from build123d import *

# Parameters (mm, degrees)
ESQUISSE1_W             = 29.88
ESQUISSE1_H             = 30
ESQUISSE1_W_2           = 30
BOSS_EXTRU_1_DEPTH      = 3
ENL_V_MAT_EXTRU_1_DEPTH = 3


with BuildPart() as part:
    # Esquisse1 → Boss.-Extru.1 (new body)
    with BuildSketch(Plane(origin=(0, 0, 0), x_dir=(0, 0, -1), z_dir=(1, 0, 0))):
        with Locations((29.757813765, -25.688259109)):
            Rectangle(ESQUISSE1_W, ESQUISSE1_H)
        with Locations((-0.182186235, -25.688259109)):
            Rectangle(ESQUISSE1_W_2, ESQUISSE1_H)
        with Locations((-0.182186235, 4.311740891)):
            Rectangle(ESQUISSE1_W_2, ESQUISSE1_H)
    extrude(amount=BOSS_EXTRU_1_DEPTH)

    # Esquisse2 → Enlèv. mat.-Extru.1 (cut)
    with BuildSketch(Plane.ZY):
        with BuildLine():
            ThreePointArc((-42.197813765, -39.188259109), (-42.273934233, -38.805575677), (-42.490706984, -38.481152328))
            Line((-42.490706984, -38.481152328), (-43.904920546, -39.89536589))
            ThreePointArc((-43.904920546, -39.89536589), (-42.815130333, -40.112138642), (-42.197813765, -39.188259109))
        make_face()
        with BuildLine():
            Line((-43.904920546, -39.89536589), (-42.490706984, -38.481152328))
            ThreePointArc((-42.490706984, -38.481152328), (-43.904920546, -38.481152328), (-43.904920546, -39.89536589))
        make_face()
        with BuildLine():
            ThreePointArc((-43.904920546, -11.481152328), (-43.904920546, -12.89536589), (-42.490706984, -12.89536589))
            Line((-42.490706984, -12.89536589), (-43.904920546, -11.481152328))
        make_face()
        with BuildLine():
            Line((-43.904920546, -11.481152328), (-42.490706984, -12.89536589))
            ThreePointArc((-42.490706984, -12.89536589), (-42.273934233, -12.570942542), (-42.197813765, -12.188259109))
            ThreePointArc((-42.197813765, -12.188259109), (-42.815130333, -11.264379577), (-43.904920546, -11.481152328))
        make_face()
        with BuildLine():
            ThreePointArc((-14.024920546, -11.481152328), (-14.024920546, -12.89536589), (-12.610706984, -12.89536589))
            Line((-12.610706984, -12.89536589), (-14.024920546, -11.481152328))
        make_face()
        with BuildLine():
            Line((-14.024920546, -11.481152328), (-12.610706984, -12.89536589))
            ThreePointArc((-12.610706984, -12.89536589), (-12.393934233, -12.570942542), (-12.317813765, -12.188259109))
            ThreePointArc((-12.317813765, -12.188259109), (-12.935130333, -11.264379577), (-14.024920546, -11.481152328))
        make_face()
        with BuildLine():
            ThreePointArc((-14.024920546, 18.518847672), (-14.024920546, 17.10463411), (-12.610706984, 17.10463411))
            Line((-12.610706984, 17.10463411), (-14.024920546, 18.518847672))
        make_face()
        with BuildLine():
            Line((-14.024920546, 18.518847672), (-12.610706984, 17.10463411))
            ThreePointArc((-12.610706984, 17.10463411), (-12.393934233, 17.429057458), (-12.317813765, 17.811740891))
            ThreePointArc((-12.317813765, 17.811740891), (-12.935130333, 18.735620423), (-14.024920546, 18.518847672))
        make_face()
        with BuildLine():
            ThreePointArc((14.389293016, 18.518847672), (12.975079454, 18.518847672), (12.975079454, 17.10463411))
            Line((12.975079454, 17.10463411), (14.389293016, 18.518847672))
        make_face()
        with BuildLine():
            Line((14.389293016, 18.518847672), (12.975079454, 17.10463411))
            ThreePointArc((12.975079454, 17.10463411), (14.064869667, 16.887861358), (14.682186235, 17.811740891))
            ThreePointArc((14.682186235, 17.811740891), (14.606065767, 18.194424323), (14.389293016, 18.518847672))
        make_face()
        with BuildLine():
            ThreePointArc((14.682186235, -39.188259109), (14.064869667, -38.264379577), (12.975079454, -38.481152328))
            Line((12.975079454, -38.481152328), (14.389293016, -39.89536589))
            ThreePointArc((14.389293016, -39.89536589), (14.606065767, -39.570942542), (14.682186235, -39.188259109))
        make_face()
        with BuildLine():
            Line((14.389293016, -39.89536589), (12.975079454, -38.481152328))
            ThreePointArc((12.975079454, -38.481152328), (12.975079454, -39.89536589), (14.389293016, -39.89536589))
        make_face()
    extrude(amount=-ENL_V_MAT_EXTRU_1_DEPTH, mode=Mode.SUBTRACT)


solid = part.part
CAD build for the part. Positions are in the model's coordinates, mm. A direction names the side the tool comes from. Give positions to 0.01 mm unless a question says otherwise; leave off trailing zeros. Order: outer loops, then holes, each group sorted by start corner. A loop starts at its lowest first (then second) coordinate and runs counter-clockwise, first axis right, second up. Notation, with made-up numbers: (46.5, 44.25) - (103.5, 44.25) arc R26 ccw to (103.5, 69.25) - close; hole circle Ø7 at (64.5, -8.5). An arc over 180 degrees is marked (long way). Write each question's results on one line, items separated by ' | '.
1. Probe L1, parallel to Z at x = 0.75, y = -5.5; L2, parallel to Y at x = 2.75, z = -20.5. List the from-to ranges inside material, lowest first. Write a range as from..to.
Calculated:
L1: z = -14.82..15.18 | L2: y = -40.69..-10.69
2. Pin check, flat tips, straight feed: pin 1 (1.5 mm diameter, centred on x = 1, y = 4.5, fed in from -Z); pin 2 (1.5 mm diameter, centred on x = 2, z = -23, fed in from +Y). Stop position of each tip, or through.
Calculated:
pin 1: stops at z = -14.82 | pin 2: stops at y = -10.69
3. 3-axis set-ups, long thin cutter, end or side, ignore diameter. For faces 1 (the face through (1, -10.688, -30)), 2 (the face through (1, -26, -44.698)): which of +Z, -Z, +X, -X, +Y, -Y reach the whole face in a straight line?
Calculated:
face 1: -Z, +X, -X, +Y | face 2: -Z, +X, -X, +Y, -Y
4. Saw through at C-C on z = -37.5. List the corners of the cut face in (x, y).
Calculated:
outline: (0, -40.69) - (3, -40.69) - (3, -10.69) - (0, -10.69) - close
5. Saw through at A-A on x = 0.85. List the corners of the cut face in (y, z).
Calculated:
outline: (-40.69, -44.7) - (-10.69, -44.7) - (-10.69, -14.82) - (19.31, -14.82) - (19.31, 15.18) - (-40.69, 15.18) - close; hole circle Ø2 at (-39.19, -43.2); hole circle Ø2 at (-39.19, 13.68); hole circle Ø2 at (-12.19, -43.2); hole circle Ø2 at (-12.19, -13.32); hole circle Ø2 at (17.81, -13.32); hole circle Ø2 at (17.81, 13.68)
6. Saw through at B-B on y = -4.5. List the corners of the cut face in (x, z).
Calculated:
outline: (0, -14.82) - (3, -14.82) - (3, 15.18) - (0, 15.18) - close
